Design review of the part built by this model. Coordinates are the model's own, in mm. A direction names the side the tool comes from. Coordinates: 2 decimals unless noted, no trailing zeros. Order: outer loops, then holes, each group sorted by start corner. A loop starts at its lowest first (then second) coordinate and runs counter-clockwise, first axis right, second up.
from build123d import *

# Parameters (mm, degrees)
SKETCH2_R            = 2.54
SKETCH2_W            = 10.16
SKETCH2_H            = 10.16
BOSS_EXTRUDE1_DEPTH  = 2.54
CUT_EXTRUDE1_DEPTH   = 0.508
CIRPATTERN1_COUNT    = 2
CIRPATTERN1_ANGLE    = 50
MIRROR2_COPY_1_DEPTH = 0.508


with BuildPart() as part:
    # Sketch2 → Boss-Extrude1 (new body)
    with BuildSketch(Plane.XY):
        with BuildLine():
            Line((-38.1, -65.991135768), (-38.1, 65.991135768))
            ThreePointArc((-38.1, 65.991135768), (0, 76.2), (38.1, 65.991135768))
            Line((38.1, 65.991135768), (38.1, -65.991135768))
            ThreePointArc((38.1, -65.991135768), (0, -76.2), (-38.1, -65.991135768))
        make_face()
        with Locations(Location((30.593335967, 65.607620704, 0), (0, 0, 180))):
            Circle(SKETCH2_R, mode=Mode.SUBTRACT)
        with Locations((-30.593335967, -65.607620704)):
            Circle(SKETCH2_R, mode=Mode.SUBTRACT)
        with Locations(Location((-30.593335967, 65.607620704, 0), (0, 0, 180))):
            Circle(SKETCH2_R, mode=Mode.SUBTRACT)
        with Locations((30.593335967, -65.607620704)):
            Circle(SKETCH2_R, mode=Mode.SUBTRACT)
        Rectangle(SKETCH2_W, SKETCH2_H, mode=Mode.SUBTRACT)
    extrude(amount=BOSS_EXTRUDE1_DEPTH)

    # Sketch6 → Cut-Extrude1 (cut)
    with BuildSketch(Plane.XY):
        with BuildLine():
            ThreePointArc((30.882724846, 69.661304223), (28.875815352, 61.924385857), (33.512622116, 68.434962986))
            ThreePointArc((33.512622116, 68.434962986), (32.203511545, 69.060653372), (30.882724846, 69.661304223))
        make_face()
    cut_extrude1 = extrude(amount=CUT_EXTRUDE1_DEPTH, mode=Mode.SUBTRACT)

    # CirPattern1: Cut-Extrude1 ×2 about axis
    cirpattern1_axis = Axis((0, 0, 2.54), (0, 0, 1))
    for i in range(1, CIRPATTERN1_COUNT):
        add(cut_extrude1.rotate(cirpattern1_axis, i * CIRPATTERN1_ANGLE / (CIRPATTERN1_COUNT - 1)), mode=Mode.SUBTRACT)

    # Mirror2: Cut-Extrude1 across plane
    add(cut_extrude1.mirror(Plane(origin=(0, 0, 0), x_dir=(0, 0, 1), z_dir=(0, -1, 0))), mode=Mode.SUBTRACT)

    # Mirror2 copy 1 sketch → Mirror2 copy 1 (cut)
    with BuildSketch(Plane(origin=(0, 0, 0), x_dir=(0.6427876096865379, -0.7660444431189793, 0), z_dir=(0, 0, 1))):
        with BuildLine():
            ThreePointArc((30.882724846, -69.661304223), (28.875815352, -61.924385857), (33.512622116, -68.434962986))
            ThreePointArc((33.512622116, -68.434962986), (32.203511545, -69.060653372), (30.882724846, -69.661304223))
        make_face()
    extrude(amount=MIRROR2_COPY_1_DEPTH, mode=Mode.SUBTRACT)


solid = part.part
1. To check wall thickness, follow line 1 (X direction, y = 3, z = 1.1); line 2 (Y direction, x = -32, z = 2.1); line 3 (Y direction, x = 28.5, z = 1.2). State the ranges of each line that lie inside material, in increasing order.
2. Add section B-B (x = 16). Give the boundary of the cut face in (y, z).
3. Add section A-A (z = 1.5). Give the boundary of the cut face in (x, y), and give its area (3 significant figures).
4. Insertion check: pin 1 (3 mm diameter, centred on x = -30.59, y = -65.61, fed in from -Z); pin 2 (13 mm diameter, centred on x = -30.59, y = 65.61, fed in from +Z); pin 3 (2.5 mm diameter, centred on x = -32, y = 65, fed in from -Z); pin 4 (1.3 mm diameter, centred on x = 2, z = 1.5, fed in from +Y). Each pin has a flat end and moves straight along its axis. Give the tip position at first contact, or say it passes through.
5. Mouldability with a two-part tool opening along X and no side actions: class faces 3 (the flat face through (9, 1, 2.54)), 4 (the cylindrical face through (-29.02, -61.86, 0.25)), 5 (the cylindrical face through (0.559, -76.198, 1.252)) as pulls with the +X half, pulls with the -X half, needs draft (parallel to the pull), parting line crosses it, or undercut.
6. For faces 1 (the cylindrical face through (-0.559, 76.198, 1.252)), 2 (the flat face through (31.4, -63, 0.508)), list the 3-axis set-ups (+Z, -Z, +X, -X, +Y, -Y) from which the entire face can be reached by the end or side of a thin tool; tool diameter is ignored.
Solution:
1. line 1: x = -38.1 to -5.08, 5.08 to 38.1
1. line 2: y = -69.16 to -67.72, -63.49 to 63.49, 67.72 to 69.16
1. line 3: y = -70.67 to -67.05, -64.17 to 64.17, 67.05 to 70.67
2. outline: (-74.5, 0) - (74.5, 0) - (74.5, 2.54) - (-74.5, 2.54) - close
3. outline: (-38.1, -65.99) arc R76.2 ccw to (38.1, -65.99) - (38.1, 65.99) arc R76.2 ccw to (-38.1, 65.99) - close; hole circle Ø5.08 at (-30.59, -65.61); hole circle Ø5.08 at (-30.59, 65.61); hole (-5.08, -5.08) - (5.08, -5.08) - (5.08, 5.08) - (-5.08, 5.08) - close; hole circle Ø5.08 at (30.59, -65.61); hole circle Ø5.08 at (30.59, 65.61)
3. area: 10,900 mm2
4. pin 1: passes through
4. pin 2: stops at z = 2.54
4. pin 3: stops at z = 0.51
4. pin 4: stops at y = 76.19
5. face 3: needs draft
5. face 4: undercut
5. face 5: parting line crosses it
6. face 1: +Z, -Z, +Y
6. face 2: -Z
